For this review, take the finished solid that the model builds, in its own axes (mm). A direction names the side the tool comes from. Give positions to 0.01 mm unless a question says otherwise; leave off trailing zeros. Order: outer loops, then holes, each group sorted by start corner. A loop starts at its lowest first (then second) coordinate and runs counter-clockwise, first axis right, second up. Notation, with made-up numbers: M 31,-36.5 L 71,-36.5 A35 ccw 71,2.5 Z; hole C -2.5,9 d3. An arc over 180 degrees is marked long. Answer as CSV lines item,"result". Start each with the question number.
1. Clearance check with flat-ended pins moving along their axes: P1, Ø1, axis at y = 0, z = -5, coming from the +X side; P2, Ø0.5, axis at x = 0.5, z = 5.5, coming from the -Y side. State where each tip first meets the part, or that it passes through.
2. We need section C-C, the plane z = -2.25. Give the boundary of the cut face in (x, y).
3. We need section D-D, the plane x = 1.8. Give the boundary of the cut face in (y, z).
4. Machinability: for faces 1 (the flat face through (0, 0, 5)), 2 (the flat face through (0, 1, 6)), 3 (the flat face through (-1, 0, -12)), which of the approach directions +Z, -Z, +X, -X, +Y, -Y give a long, thin tool a straight path to every point of the face, cutting with its end or side? Answer none if there is none.
5. We need section A-A, the plane x = 0. Give the boundary of the cut face in (y, z).
6. For line 1 along Z through (x, y) = (-1.7, 1.25); line 2 along X through (y, z) = (0.1, 2.75); line 3 along Z through (x, y) = (-0.45, -0.8), list the stretches that pass through material, from the lowest coordinate up.
7. Mouldability with a two-part tool opening along Y and no side actions: class faces 4 (the cylindrical face through (2.385, 0.751, 2.958)), 5 (the flat face through (0, -0.5, 5.5)), 6 (the flat face through (0, -1, 6)) as pulls with the +Y half, pulls with the -Y half, needs draft (parallel to the pull), parting line crosses it, or undercut.
8. We need section B-B, the plane y = 0.7. Give the boundary of the cut face in (x, z).
from build123d import *

# Parameters (mm, degrees)
SKETCH1_R           = 2.5
BOSS_EXTRUDE1_DEPTH = 6
SKETCH2_W           = 5.368595506
SKETCH2_H           = 1
CUT_EXTRUDE1_DEPTH  = 1
SKETCH3_R           = 1.5
BOSS_EXTRUDE2_DEPTH = 12
SKETCH4_R           = 0.5
BOSS_EXTRUDE3_DEPTH = 4
BOSS_EXTRUDE3_TAPER = 3


with BuildPart() as part:
    # Sketch1 → Boss-Extrude1 (new body)
    with BuildSketch(Plane.XY):
        Circle(SKETCH1_R)
    extrude(amount=BOSS_EXTRUDE1_DEPTH)

    # Sketch2 → Cut-Extrude1 (cut)
    with BuildSketch(Plane.XY.offset(6)):
        Rectangle(SKETCH2_W, SKETCH2_H)
    extrude(amount=-CUT_EXTRUDE1_DEPTH, mode=Mode.SUBTRACT)

    # Sketch3 → Boss-Extrude2 (add)
    with BuildSketch(Plane(origin=(0, 0, 0), x_dir=(-1, 0, 0), z_dir=(0, 0, -1))):
        Circle(SKETCH3_R)
    extrude(amount=BOSS_EXTRUDE2_DEPTH)

    # Sketch4 → Boss-Extrude3 (add)
    with BuildSketch(Plane(origin=(0, 0, -12), x_dir=(-1, 0, 0), z_dir=(0, 0, -1))):
        Circle(SKETCH4_R)
    extrude(amount=BOSS_EXTRUDE3_DEPTH, taper=BOSS_EXTRUDE3_TAPER)


solid = part.part
Result set:
1,P1,"x = 1.5"
1,P2,"y = -2.49"
2,outline,"C 0,0 d3"
3,outline,"M -1.73,0 L 1.73,0 L 1.73,6 L 0.5,6 L 0.5,5 L -0.5,5 L -0.5,6 L -1.73,6 Z"
4,face 1,"+Z, +X, -X"
4,face 2,"+Z, +X, -X, +Y, -Y"
4,face 3,"-Z"
5,outline,"M -2.5,0 L -1.5,0 L -1.5,-12 L -0.5,-12 L -0.29,-16 L 0.29,-16 L 0.5,-12 L 1.5,-12 L 1.5,0 L 2.5,0 L 2.5,6 L 0.5,6 L 0.5,5 L -0.5,5 L -0.5,6 L -2.5,6 Z"
6,line 1,"0 to 6"
6,line 2,"-2.5 to 2.5"
6,line 3,"-12 to 6"
7,face 4,"parting line crosses it"
7,face 5,"undercut"
7,face 6,"needs draft"
8,outline,"M -2.4,0 L -1.33,0 L -1.33,-12 L 1.33,-12 L 1.33,0 L 2.4,0 L 2.4,6 L -2.4,6 Z"
